Can you work these out from the model? Positions are in its coordinate system, mm. Face numbers are marked on the shaded views. A direction names the side the tool comes from. Round coordinates to 2 decimals unless told otherwise and drop trailing zeros. Write each loop counter-clockwise with the first axis right and the second up, starting at its lowest first coordinate (ties: lowest second). Pieces come first, ordered by that corner, then holes. Notation, with made-up numbers: (88, -33) -> (128, -33) arc R13 ccw to (128, -15) -> close; hole circle Ø9 at (81, -20.5). An arc over 180 degrees is marked (long way). Write item = value, one per line. Start each with the question number.
1) Imagine slicing it at D-D, the plane x = -17. Please give me the cut outline in (y, z).
2) For the marked faces 1 and 2, which set-ups out of +Z, -Z, +X, -X, +Y, -Y let a thin tool reach every point of the face, with its end or its side?
3) Imagine slicing it at C-C, the plane z = -33. Please give me the cut outline in (x, y).
4) If I drill on line 1 (Z direction, x = 6, y = -15.5); line 2 (X direction, y = -13, z = -43.5); line 3 (Y direction, x = 8.5, z = -59.5), over which ranges is the centre line in solid material (lowest first)?
5) Imagine slicing it at B-B, the plane y = 11. Please give me the cut outline in (x, z).
6) I'm going to push flat-ended pins straight in: pin 1 (1 mm diameter, centred on y = -1, z = -80.5, fed in from -X); pin 2 (10 mm diameter, centred on y = 17.5, z = -88, fed in from +X); pin 3 (6 mm diameter, centred on y = -15, z = -68.5, fed in from +X). Where does each tip first touch, or does it pass through?
7) Imagine slicing it at A-A, the plane x = 0. Please give me the cut outline in (y, z).
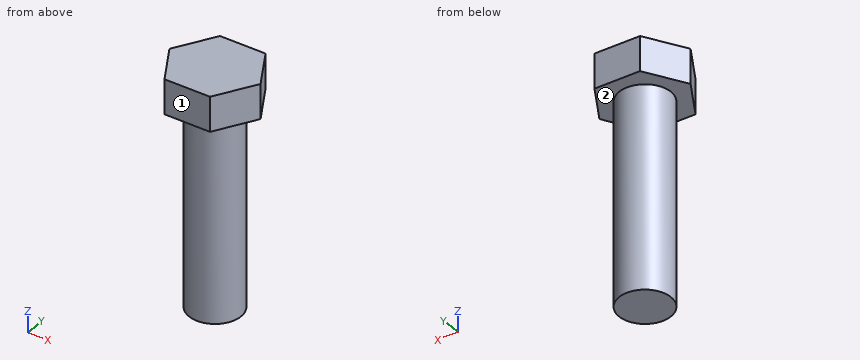
from build123d import *

# Parameters (mm, degrees)
BOSS_EXTRUDE1_DEPTH = 20
SKETCH2_R           = 15
BOSS_EXTRUDE2_DEPTH = 117


with BuildPart() as part:
    # Sketch1 → Boss-Extrude1 (new body)
    with BuildSketch(Plane.XY):
        Polygon((26.558112383, 0), (13.279056191, 23), (-13.279056191, 23), (-26.558112383, 0), (-13.279056191, -23), (13.279056191, -23), align=None)
    extrude(amount=-BOSS_EXTRUDE1_DEPTH)

    # Sketch2 → Boss-Extrude2 (add)
    with BuildSketch(Plane(origin=(0, 0, -20), x_dir=(-1, 0, 0), z_dir=(0, 0, -1))):
        Circle(SKETCH2_R)
    extrude(amount=BOSS_EXTRUDE2_DEPTH)


solid = part.part
Reported:
q1.outline = (-16.56, -20) -> (16.56, -20) -> (16.56, 0) -> (-16.56, 0) -> close
q2.face_1 = +Z, -Z, +X, -X, -Y
q2.face_2 = -Z
q3.outline = circle Ø30 at (0, 0)
q4.line_1 = -20 to 0
q4.line_2 = -7.48 to 7.48
q4.line_3 = -12.36 to 12.36
q5.outline = (-20.21, -20) -> (-10.2, -20) -> (-10.2, -137) -> (10.2, -137) -> (10.2, -20) -> (20.21, -20) -> (20.21, 0) -> (-20.21, 0) -> close
q6.pin_1 = -14.99
q6.pin_2 = 8.29
q6.pin_3 = 9
q7.outline = (-23, -20) -> (-15, -20) -> (-15, -137) -> (15, -137) -> (15, -20) -> (23, -20) -> (23, 0) -> (-23, 0) -> close
